Could you check a few things on this model? Use its own coordinates, in mm. A direction names the side the tool comes from. Coordinates: 2 decimals unless noted, no trailing zeros. Write each loop counter-clockwise with the first axis right and the second up, starting at its lowest first coordinate (ties: lowest second). Pieces come first, ordered by that corner, then holes. Notation, with made-up numbers: (39.25, 22.25) - (85.25, 22.25) arc R21 cw to (85.25, 26.25) - close; hole circle Ø4 at (30, 60.5). An arc over 180 degrees is marked (long way). Answer as a JSON object with one key per item and string values. Group by question number.
1) On a 3-axis mill with a long thin cutter (end or side, diameter ignored), from which of +Z, -Z, +X, -X, +Y, -Y can I reach the whole of each face in a straight line? I mean faces 1 (the flat face through (-4, 59.69, 3)), 2 (the flat face through (-2.348, 53.429, -4.144)), 3 (the flat face through (0, 59.69, 5)), 4 (the cylindrical face through (-3.78, 63.45, 2.9)), 5 (the flat face through (4, 59.69, 3)). Say none if no direction works.
2) Please list where these lines run through material, in increasing order: line 1 along Y through (x, z) = (5.5, 0.5); line 2 along X through (y, z) = (52.5, 2); line 3 along Z through (x, y) = (-2.75, 26).
3) If we section it at B-B (x = -1.5): Write out the boundary of the cut face in (y, z), plus the area to 3 significant figures.
4) Will these pins go through, and if not, where does the flat tip stop? pin 1 Ø5 at (x, y) = (-4, 50) entering from +Z; pin 2 Ø1.5 at (x, y) = (5, 27.5) entering from -Z; pin 3 Ø2.5 at (y, z) = (54.5, 0) entering from +X.
5) If we section it at C-C (y = 56): Write out the boundary of the cut face in (x, z).
6) If we section it at A-A (z = -0.75): Write out the boundary of the cut face in (x, y), plus the area to 3 significant figures.
```python
from build123d import *

# Parameters (mm, degrees)
BOSS_EXTRUDE1_DEPTH = 59.69
SKETCH2_R           = 4.7625
BOSS_EXTRUDE2_DEPTH = 67.31
CUT_EXTRUDE1_DEPTH  = 12.7


with BuildPart() as part:
    # Sketch1 → Boss-Extrude1 (new body)
    with BuildSketch(Plane(origin=(0, 0, 0), x_dir=(1, 0, 0), z_dir=(0, 1, 0))):
        Polygon((6.35, -3.666174209), (6.35, 3.666174209), (0, 7.332348419), (-6.35, 3.666174209), (-6.35, -3.666174209), (0, -7.332348419), align=None)
    extrude(amount=BOSS_EXTRUDE1_DEPTH)

    # Sketch2 → Boss-Extrude2 (add)
    with BuildSketch(Plane(origin=(0, 0, 0), x_dir=(1, 0, 0), z_dir=(0, 1, 0))):
        Circle(SKETCH2_R)
    extrude(amount=BOSS_EXTRUDE2_DEPTH)

    # Sketch3 → Cut-Extrude1 (cut)
    with BuildSketch(Plane(origin=(0, 59.69, 0), x_dir=(1, 0, 0), z_dir=(0, 1, 0))):
        Polygon((0, -7.332348419), (6.35, -3.666174209), (6.35, 3.666174209), (0, 7.332348419), (-6.35, 3.666174209), (-6.35, -3.666174209), align=None)
        Polygon((4.7625, -2.749630657), (4.7625, 2.749630657), (0, 5.499261314), (-4.7625, 2.749630657), (-4.7625, -2.749630657), (0, -5.499261314), align=None, mode=Mode.SUBTRACT)
    extrude(amount=-CUT_EXTRUDE1_DEPTH, mode=Mode.SUBTRACT)


solid = part.part
```
Here are the results:
{
 "1": {"face 1": "+Z, -X, +Y", "face 2": "-Z, -X, +Y", "face 3": "+Z, +Y", "face 4": "+Y", "face 5": "+Z, +X, +Y"},
 "2": {"line 1": "y = 0 to 46.99", "line 2": "x = -4.76 to 4.76", "line 3": "z = -5.74 to 5.74"},
 "3": {"outline": "(0, -6.47) - (46.99, -6.47) - (46.99, -4.63) - (59.69, -4.63) - (59.69, -4.52) - (67.31, -4.52) - (67.31, 4.52) - (59.69, 4.52) - (59.69, 4.63) - (46.99, 4.63) - (46.99, 6.47) - (0, 6.47) - close", "area": "794 mm²"},
 "4": {"pin 1": "stops at z = 4.63", "pin 2": "stops at z = -4.88", "pin 3": "stops at x = 4.76"},
 "5": {"outline": "(-4.76, -2.75) - (0, -5.5) - (4.76, -2.75) - (4.76, 2.75) - (0, 5.5) - (-4.76, 2.75) - close"},
 "6": {"outline": "(-6.35, 0) - (6.35, 0) - (6.35, 46.99) - (4.76, 46.99) - (4.76, 59.69) - (4.7, 59.69) - (4.7, 67.31) - (-4.7, 67.31) - (-4.7, 59.69) - (-4.76, 59.69) - (-4.76, 46.99) - (-6.35, 46.99) - close", "area": "789 mm²"}
}
